Work out the finished part from the listing and answer in its coordinate system (mm). A direction names the side the tool comes from. Coordinates: 2 decimals unless noted, no trailing zeros. Order: outer loops, then holes, each group sorted by start corner. A loop starts at its lowest first (then second) coordinate and runs counter-clockwise, first axis right, second up. Notation, with made-up numbers: M 79,50 L 133,50 A26 cw 133,64 Z; hole C 22.5,81 d8. An arc over 180 degrees is marked long. Use a Markdown table: item, result.
from build123d import *

# Parameters (mm, degrees)
SKETCH1_R           = 4.5
BOSS_EXTRUDE1_DEPTH = 9.5
BOSS_EXTRUDE2_DEPTH = 19.88
BOSS_EXTRUDE3_DEPTH = 7.72
SKETCH5_R           = 1.55
CUT_EXTRUDE1_DEPTH  = 7.5
SKETCH6_R           = 11
BOSS_EXTRUDE4_DEPTH = 2
BOSS_EXTRUDE5_DEPTH = 22
CHAMFER1_SIZE       = 0.2
FILLET1_R           = 0.5
FILLET2_R           = 0.7
CHAMFER2_SIZE       = 0.5
FILLET3_R           = 1.5


with BuildPart() as part:
    # Sketch1 → Boss-Extrude1 (new body)
    with BuildSketch(Plane(origin=(0, 0, 0), x_dir=(1, 0, 0), z_dir=(0, 1, 0))):
        Polygon((-42, 36), (-36, 42), (-6, 42), (0, 36), (0, 6), (-6, 0), (-36, 0), (-42, 6), (-42, 12.75), (-47.25, 12.75), (-47.25, 29.25), (-42, 29.25), align=None)
        with Locations(Location((-21, 21, 0), (0, 0, 270))):
            Circle(SKETCH1_R, mode=Mode.SUBTRACT)
    extrude(amount=BOSS_EXTRUDE1_DEPTH)

    # Sketch2 → Boss-Extrude2 (add)
    with BuildSketch(Plane(origin=(0, 9.5, 0), x_dir=(1, 0, 0), z_dir=(0, 1, 0))):
        Polygon((-33, 42), (-9, 42), (0, 33), (0, 9), (-9, 0), (-33, 0), (-42, 9), (-42, 33), align=None)
    extrude(amount=BOSS_EXTRUDE2_DEPTH)

    # Sketch3 → Boss-Extrude3 (add)
    with BuildSketch(Plane(origin=(0, 29.38, 0), x_dir=(1, 0, 0), z_dir=(0, 1, 0))):
        Polygon((-42, 6), (-42, 36), (-36, 42), (-6, 42), (0, 36), (0, 6), (-6, 0), (-36, 0), align=None)
    extrude(amount=BOSS_EXTRUDE3_DEPTH)

    # Sketch5 → Cut-Extrude1 (cut)
    with BuildSketch(Plane(origin=(0, 37.1, 0), x_dir=(1, 0, 0), z_dir=(0, 1, 0))):
        with Locations(Location((-36.5, 5.5, 0), (0, 0, 270))):
            Circle(SKETCH5_R)
        with Locations(Location((-5.5, 36.5, 0), (0, 0, 270))):
            Circle(SKETCH5_R)
        with Locations(Location((-36.5, 36.5, 0), (0, 0, 270))):
            Circle(SKETCH5_R)
        with Locations(Location((-5.5, 5.5, 0), (0, 0, 270))):
            Circle(SKETCH5_R)
    extrude(amount=-CUT_EXTRUDE1_DEPTH, mode=Mode.SUBTRACT)

    # Sketch6 → Boss-Extrude4 (add)
    with BuildSketch(Plane(origin=(0, 37.1, 0), x_dir=(1, 0, 0), z_dir=(0, 1, 0))):
        with Locations(Location((-21, 21, 0), (0, 0, 270))):
            Circle(SKETCH6_R)
    extrude(amount=BOSS_EXTRUDE4_DEPTH)

    # Sketch7 → Boss-Extrude5 (add)
    with BuildSketch(Plane(origin=(0, 39.1, 0), x_dir=(1, 0, 0), z_dir=(0, 1, 0))):
        with BuildLine():
            Line((-22.5, 23), (-19.5, 23))
            ThreePointArc((-19.5, 23), (-21, 18.5), (-22.5, 23))
        make_face()
    extrude(amount=BOSS_EXTRUDE5_DEPTH)

    # Chamfer1
    chamfer1_edges = [part.edges().sort_by_distance(p)[0] for p in [
        (-5.5, 37.1, -38.05),
        (-36.5, 37.1, -7.05),
        (-5.5, 37.1, -7.05),
        (-36.5, 37.1, -38.05),
    ]]
    chamfer(chamfer1_edges, length=CHAMFER1_SIZE)

    # Fillet1
    fillet1_edges = [part.edges().sort_by_distance(p)[0] for p in [
        (-42, 4.75, -12.75),
        (-42, 4.75, -29.25),
        (-44.625, 9.5, -12.75),
        (-44.625, 9.5, -29.25),
        (-42, 9.5, -21),
        (-47.25, 4.75, -29.25),
        (-47.25, 9.5, -21),
        (-47.25, 4.75, -12.75),
        (-21, 0, -25.5),
        (-44.625, 0, -29.25),
        (-47.25, 0, -21),
        (-44.625, 0, -12.75),
        (-42, 0, -9.375),
        (-39, 0, -3),
        (-21, 0, 0),
        (-3, 0, -3),
        (0, 0, -21),
        (-3, 0, -39),
        (-21, 0, -42),
        (-39, 0, -39),
        (-42, 0, -32.625),
        (-6, 4.75, -42),
        (0, 4.75, -36),
        (-42, 4.75, -36),
        (-36, 4.75, -42),
        (0, 4.75, -6),
        (-6, 4.75, 0),
        (-36, 4.75, 0),
        (-42, 4.75, -6),
        (-42, 33.24, -36),
        (-39, 37.1, -39),
        (-36, 33.24, -42),
        (-21, 37.1, -42),
        (-6, 33.24, -42),
        (0, 33.24, -36),
        (0, 37.1, -21),
        (-3, 37.1, -39),
        (0, 33.24, -6),
        (-6, 33.24, 0),
        (-42, 33.24, -6),
        (-36, 33.24, 0),
        (-3, 37.1, -3),
        (-21, 37.1, 0),
        (-39, 37.1, -3),
        (-42, 37.1, -21),
    ]]
    fillet(fillet1_edges, radius=FILLET1_R)

    # Fillet2
    fillet2_edges = [part.edges().sort_by_distance(p)[0] for p in [
        (-21, 37.1, -32),
    ]]
    fillet(fillet2_edges, radius=FILLET2_R)

    # Chamfer2
    chamfer2_edges = [part.edges().sort_by_distance(p)[0] for p in [
        (-21, 61.1, -18.5),
    ]]
    chamfer(chamfer2_edges, length=CHAMFER2_SIZE - 0.0001)  # a hair under: the kernel refuses the full size

    # Fillet3
    fillet3_edges = [part.edges().sort_by_distance(p)[0] for p in [
        (-33, 19.44, -42),
        (-42, 19.44, -33),
        (-42, 19.44, -9),
        (-33, 19.44, 0),
        (-9, 19.44, 0),
        (0, 19.44, -9),
        (0, 19.44, -33),
        (-9, 19.44, -42),
    ]]
    fillet(fillet3_edges, radius=FILLET3_R)


solid = part.part
1. Find the intervals of material crossed by probe 1 along X at (y, z) = (33, -36.5); probe 2 along X at (y, z) = (31, -36); probe 3 along Y at (x, z) = (-4, -3.5), in increasing order.
Answers below:
| item | result |
|---|---|
| probe 1 | -41.5 to -38.05, -34.95 to -7.05, -3.95 to -0.5 |
| probe 2 | -41.96 to -37.97, -35.03 to -6.97, -4.03 to -0.04 |
| probe 3 | 0 to 9.5, 29.38 to 37.1 |
2. Section B-B on y = 11 is taken. Determine the outline of the cut face in (x, z).
Answers below:
| item | result |
|---|---|
| outline | M -42,-32.38 A1.5 ccw -41.56,-33.44 L -33.44,-41.56 A1.5 ccw -32.38,-42 L -9.62,-42 A1.5 ccw -8.56,-41.56 L -0.44,-33.44 A1.5 ccw 0,-32.38 L 0,-9.62 A1.5 ccw -0.44,-8.56 L -8.56,-0.44 A1.5 ccw -9.62,0 L -32.38,0 A1.5 ccw -33.44,-0.44 L -41.56,-8.56 A1.5 ccw -42,-9.62 Z |
3. Flat-ended cylindrical pins translate along their axes: P1, Ø8, axis at x = -21, z = -7, coming from the +Y side; P2, Ø2, axis at x = -44.5, y = 4.5, coming from the -Z side; P3, Ø4, axis at x = -19.5, z = -5.5, coming from the +Y side; P4, Ø4, axis at x = -9.5, y = 41.5, coming from the +Z side. Find the tip coordinate at first contact, or state that the pin passes through.
Answers below:
| item | result |
|---|---|
| P1 | y = 39.1 |
| P2 | z = -29.25 |
| P3 | y = 37.1 |
| P4 | through |
4. For faces 4 (the face through (-3, 9.5, -38)), 5 (the face through (-37, 19, -4)), 6 (the face through (-5.034, 33.301, -35.022)), determine the directions among +Z, -Z, +X, -X, +Y, -Y from which every point of the face is accessible in a straight line to the end or side of a thin tool.
Answers below:
| item | result |
|---|---|
| face 4 | -Z, +X |
| face 5 | +Z, -X |
| face 6 | +Y |
5. For a pull along Z with two mould halves and no side action, classify faces 1 (the face through (-36, 29.6, -37)), 2 (the face through (-3.15, 36.96, -3.07)), 3 (the face through (-21, 61.1, -21)) as +Z half, -Z half, draft (parallel to the pull), parting line (faces both ways), or undercut.
Answers below:
| item | result |
|---|---|
| face 1 | undercut |
| face 2 | +Z half |
| face 3 | draft |
